from build123d import *

# Parameters (mm, degrees)
ESBO_O1_W                = 42
ESBO_O1_H                = 42
RESSALTO_EXTRUS_O3_DEPTH = 6
ESBO_O7_W                = 42
ESBO_O7_H                = 11
RESSALTO_EXTRUS_O4_DEPTH = 10
CORTE_EXTRUS_O3_REACH    = 35.734
ESBO_O6_R                = 11
ESBO_O6_R_2              = 1.75
CHANFRO1_SIZE            = 4
FILETE1_R                = 2.5
ESBO_O8_R                = 2.25
CORTE_EXTRUS_O4_DEPTH    = 11
ESBO_O9_R                = 3
CORTE_EXTRUS_O5_DEPTH    = 10
CORTE_EXTRUS_O6_REACH    = 42.719
ESBO_O10_R               = 4.25


with BuildPart() as part:
    # Esboço1 → Ressalto-extrusão3 (new body)
    with BuildSketch(Plane.XY):
        Rectangle(ESBO_O1_W, ESBO_O1_H)
    extrude(amount=RESSALTO_EXTRUS_O3_DEPTH)

    # Esboço7 → Ressalto-extrusão4 (add)
    with BuildSketch(Plane.XY.offset(6)):
        with Locations((0, -15.5)):
            Rectangle(ESBO_O7_W, ESBO_O7_H)
    extrude(amount=RESSALTO_EXTRUS_O4_DEPTH)

    # Corte-extrusão3: up to this face of the body (flat: up to its plane)
    corte_extrus_o3_end = Plane(part.part.faces().sort_by_distance((0, -15.5, 16))[0])
    # Esboço6 → Corte-extrusão3 (cut, up to the picked face)
    with BuildSketch(Plane(origin=(0, 0, 0), x_dir=(-1, 0, 0), z_dir=(0, 0, -1)), mode=Mode.PRIVATE) as corte_extrus_o3_sk1:
        Circle(ESBO_O6_R)
    corte_extrus_o3_tool1 = split(extrude(corte_extrus_o3_sk1.sketch, amount=-CORTE_EXTRUS_O3_REACH, mode=Mode.PRIVATE), bisect_by=corte_extrus_o3_end, keep=Keep.BOTH, mode=Mode.PRIVATE)
    # Esboço6 → Corte-extrusão3 (cut, up to the picked face)
    with BuildSketch(Plane(origin=(0, 0, 0), x_dir=(-1, 0, 0), z_dir=(0, 0, -1)), mode=Mode.PRIVATE) as corte_extrus_o3_sk2:
        with Locations((-15.5, 15.5)):
            Circle(ESBO_O6_R_2)
    corte_extrus_o3_tool2 = split(extrude(corte_extrus_o3_sk2.sketch, amount=-CORTE_EXTRUS_O3_REACH, mode=Mode.PRIVATE), bisect_by=corte_extrus_o3_end, keep=Keep.BOTH, mode=Mode.PRIVATE)
    # Esboço6 → Corte-extrusão3 (cut, up to the picked face)
    with BuildSketch(Plane(origin=(0, 0, 0), x_dir=(-1, 0, 0), z_dir=(0, 0, -1)), mode=Mode.PRIVATE) as corte_extrus_o3_sk3:
        with Locations((15.5, 15.5)):
            Circle(ESBO_O6_R_2)
    corte_extrus_o3_tool3 = split(extrude(corte_extrus_o3_sk3.sketch, amount=-CORTE_EXTRUS_O3_REACH, mode=Mode.PRIVATE), bisect_by=corte_extrus_o3_end, keep=Keep.BOTH, mode=Mode.PRIVATE)
    # Esboço6 → Corte-extrusão3 (cut, up to the picked face)
    with BuildSketch(Plane(origin=(0, 0, 0), x_dir=(-1, 0, 0), z_dir=(0, 0, -1)), mode=Mode.PRIVATE) as corte_extrus_o3_sk4:
        with Locations((15.5, -15.5)):
            Circle(ESBO_O6_R_2)
    corte_extrus_o3_tool4 = split(extrude(corte_extrus_o3_sk4.sketch, amount=-CORTE_EXTRUS_O3_REACH, mode=Mode.PRIVATE), bisect_by=corte_extrus_o3_end, keep=Keep.BOTH, mode=Mode.PRIVATE)
    # Esboço6 → Corte-extrusão3 (cut, up to the picked face)
    with BuildSketch(Plane(origin=(0, 0, 0), x_dir=(-1, 0, 0), z_dir=(0, 0, -1)), mode=Mode.PRIVATE) as corte_extrus_o3_sk5:
        with Locations((-15.5, -15.5)):
            Circle(ESBO_O6_R_2)
    corte_extrus_o3_tool5 = split(extrude(corte_extrus_o3_sk5.sketch, amount=-CORTE_EXTRUS_O3_REACH, mode=Mode.PRIVATE), bisect_by=corte_extrus_o3_end, keep=Keep.BOTH, mode=Mode.PRIVATE)
    add(corte_extrus_o3_tool1.solids().sort_by(Axis((0, 0, 0), (0, 0, 1)))[0], mode=Mode.SUBTRACT)
    add(corte_extrus_o3_tool2.solids().sort_by(Axis((15.5, 15.5, 0), (0, 0, 1)))[0], mode=Mode.SUBTRACT)
    add(corte_extrus_o3_tool3.solids().sort_by(Axis((-15.5, 15.5, 0), (0, 0, 1)))[0], mode=Mode.SUBTRACT)
    add(corte_extrus_o3_tool4.solids().sort_by(Axis((-15.5, -15.5, 0), (0, 0, 1)))[0], mode=Mode.SUBTRACT)
    add(corte_extrus_o3_tool5.solids().sort_by(Axis((15.5, -15.5, 0), (0, 0, 1)))[0], mode=Mode.SUBTRACT)

    # Chanfro1
    chanfro1_edges = [part.edges().sort_by_distance(p)[0] for p in [
        (-21, 21, 3),
        (21, 21, 3),
    ]]
    chamfer(chanfro1_edges, length=CHANFRO1_SIZE)

    # Filete1
    filete1_edges = [part.edges().sort_by_distance(p)[0] for p in [
        (12.791287847, -10, 6),
        (-12.791287847, -10, 6),
    ]]
    fillet(filete1_edges, radius=FILETE1_R)

    # Esboço8 → Corte-extrusão4 (cut)
    with BuildSketch(Plane.XZ.offset(21)):
        with Locations((-10, 11)):
            Circle(ESBO_O8_R)
        with Locations((10, 11)):
            Circle(ESBO_O8_R)
    extrude(amount=-CORTE_EXTRUS_O4_DEPTH, mode=Mode.SUBTRACT)

    # Esboço9 → Corte-extrusão5 (cut)
    with BuildSketch(Plane.XY.offset(16)):
        with Locations((-15.5, -15.5)):
            Circle(ESBO_O9_R)
        with Locations((15.5, -15.5)):
            Circle(ESBO_O9_R)
    extrude(amount=-CORTE_EXTRUS_O5_DEPTH, mode=Mode.SUBTRACT)

    # Esboço10 → Corte-extrusão6 (cut, up to next)
    with BuildSketch(Plane(origin=(0, -10, 0), x_dir=(1, 0, 0), z_dir=(0, 1, 0)), mode=Mode.PRIVATE) as corte_extrus_o6_sk1:
        with Locations((10, -11)):
            Circle(ESBO_O10_R)
    corte_extrus_o6_tool1 = extrude(corte_extrus_o6_sk1.sketch, amount=CORTE_EXTRUS_O6_REACH, mode=Mode.PRIVATE) & part.part
    # Esboço10 → Corte-extrusão6 (cut, up to next)
    with BuildSketch(Plane(origin=(0, -10, 0), x_dir=(1, 0, 0), z_dir=(0, 1, 0)), mode=Mode.PRIVATE) as corte_extrus_o6_sk2:
        with Locations((-10, -11)):
            Circle(ESBO_O10_R)
    corte_extrus_o6_tool2 = extrude(corte_extrus_o6_sk2.sketch, amount=CORTE_EXTRUS_O6_REACH, mode=Mode.PRIVATE) & part.part
    add(corte_extrus_o6_tool1.solids().sort_by_distance((10, -10, 11))[0], mode=Mode.SUBTRACT)
    add(corte_extrus_o6_tool2.solids().sort_by_distance((-10, -10, 11))[0], mode=Mode.SUBTRACT)


solid = part.part
For this review, take the finished solid that the model builds, in its own axes (mm). A direction names the side the tool comes from. Round coordinates to 2 decimals unless told otherwise and drop trailing zeros. Loops run counter-clockwise (first coordinate to the right, second up) from the corner with the lowest first, then second, coordinate; pieces in that order, holes last. Notation, with made-up numbers: (1.5, -9.75) - (32.5, -9.75) arc R19 cw to (32.5, 7.25) - close; hole circle Ø11 at (72.5, 34). An arc over 180 degrees is marked (long way). One line per question, with ' | ' between items.
Q1. Take a section at A-A (z = 11). Give the boundary of the cut face in (x, y), and give its area (3 significant figures).
Taken from the geometry:
outline: (-21, -21) - (-12.25, -21) - (-12.25, -10) - (-21, -10) - close; (-7.75, -21) - (7.75, -21) - (7.75, -10) - (4.58, -10) arc R11 cw to (-4.58, -10) - (-7.75, -10) - close; (12.25, -21) - (21, -21) - (21, -10) - (12.25, -10) - close; hole circle Ø6 at (-15.5, -15.5); hole circle Ø6 at (15.5, -15.5) | area: 300 mm²
Q2. For pin 1 (7.5 mm diameter, centred on x = -15, z = 11, fed in from +Y); pin 2 (3 mm diameter, centred on x = -7, y = 14.5, fed in from +Z); pin 3 (1.5 mm diameter, centred on x = 0, z = 13, fed in from +Y), all flat-tipped, find the tip position at first contact; note any pin that passes through.
Taken from the geometry:
pin 1: stops at y = -9.67 | pin 2: stops at z = 6 | pin 3: stops at y = -10.97
Q3. Take a section at C-C (y = -15.5). Give the boundary of the cut face in (x, z).
Taken from the geometry:
outline: (-21, 0) - (-17.25, 0) - (-17.25, 6) - (-18.5, 6) - (-18.5, 16) - (-21, 16) - close; (-13.75, 0) - (13.75, 0) - (13.75, 6) - (12.5, 6) - (12.5, 16) - (-12.5, 16) - (-12.5, 6) - (-13.75, 6) - close; (17.25, 0) - (21, 0) - (21, 16) - (18.5, 16) - (18.5, 6) - (17.25, 6) - close; hole circle Ø4.5 at (-10, 11); hole circle Ø4.5 at (10, 11)
Q4. Take a section at D-D (y = 15.5). Give the boundary of the cut face in (x, z).
Taken from the geometry:
outline: (-21, 0) - (-17.25, 0) - (-17.25, 6) - (-21, 6) - close; (-13.75, 0) - (13.75, 0) - (13.75, 6) - (-13.75, 6) - close; (17.25, 0) - (21, 0) - (21, 6) - (17.25, 6) - close
Q5. Tool access review of faces 4 (the cylindrical face through (13.1, -17.3, 11.1)), 5 (the cylindrical face through (2.38, -10.74, 4.33)), 6 (the flat face through (-19, 19, 3)), 7 (the cylindrical face through (-9.94, -9.73, 6.75)), 8 (the flat face through (0, 13, 6)): name each direction out of +Z, -Z, +X, -X, +Y, -Y from which nothing blocks a thin tool from reaching the whole face with its end or side.
Taken from the geometry:
face 4: +Z | face 5: +Z, -Z | face 6: +Z, -Z, -X, +Y | face 7: +Z, +Y | face 8: +Z, +X, -X, +Y
Q6. The part is to be moulded in two halves that separate along X. For faces 1 (the flat face through (19, 19, 3)), 2 (the cylindrical face through (-16.15, -18.43, 11.07)), 3 (the flat face through (0, 21, 3)), say which applies: released by +X, released by -X, zero draft, split by the parting line, or undercut.
Taken from the geometry:
face 1: released by +X | face 2: undercut | face 3: zero draft
Q7. For line 1 along X through (y, z) = (-17.5, 13.75); line 2 along X through (y, z) = (-14.5, 7); line 3 along Y through (x, z) = (0, 3.5), list the stretches that pass through material, from the lowest coordinate up. Write a range as [from, to].
Taken from the geometry:
line 1: x = [-21, -17.74], [-13.26, 13.26], [17.74, 21] | line 2: x = [-21, -18.33], [-12.67, 12.67], [18.33, 21] | line 3: y = [-21, -11], [11, 21]
Q8. Take a section at B-B (x = 15.5). Give the boundary of the cut face in (y, z), and give its area (3 significant figures).
Taken from the geometry:
outline: (-21, 0) - (-17.25, 0) - (-17.25, 6) - (-18.5, 6) - (-18.5, 16) - (-21, 16) - close; (-13.75, 0) - (13.75, 0) - (13.75, 6) - (-7.5, 6) arc R2.5 cw to (-10, 8.5) - (-10, 16) - (-12.5, 16) - (-12.5, 6) - (-13.75, 6) - close; (17.25, 0) - (21, 0) - (21, 6) - (17.25, 6) - close | area: 261 mm²
